from build123d import *

# Parameters (mm, degrees)
F2_R     = 1.5875
F3_DEPTH = 12.7
F4_SIZE  = 1.5875


with BuildPart() as f1:
    # F0 (on Front) → F1 (revolve)
    with BuildSketch(Plane.XZ):
        Polygon((1.27, 12.7), (0, 12.7), (-1.27, 12.7), (-1.27, 19.05), (-2.8575, 19.05), (-5.08, 6.35), (-5.08, 0), (5.08, 0), (5.08, 6.35), (2.8575, 19.05), (1.27, 19.05), align=None)
    revolve(axis=Axis((0, 0, 0), (-1, 0, 0)))

    # F2 (on Right) → F3 (cut, symmetric)
    with BuildSketch(Plane.YZ):
        Circle(F2_R)
    extrude(amount=F3_DEPTH, both=True, mode=Mode.SUBTRACT)

    # F4
    f4_edges = [f1.edges().sort_by_distance(p)[0] for p in [
        (5.08, -1.5875, 0),
        (-5.08, -1.5875, 0),
    ]]
    chamfer(f4_edges, length=F4_SIZE)


solid = f1.part
Geometry: final body of the model. Coordinates: model frame, mm. A direction names the side the tool comes from. Round coordinates to 2 decimals unless told otherwise and drop trailing zeros. Loops run counter-clockwise (first coordinate to the right, second up) from the corner with the lowest first, then second, coordinate; pieces in that order, holes last. Notation, with made-up numbers: M -18,68.5 L 6,68.5 A34 ccw 6,102.5 Z; hole C 71.25,30.25 d4. An arc over 180 degrees is marked long. Put each result on its own line as item: value. Start each with the question number.
(1) Material intervals for line 1 along X through (y, z) = (15, -11); line 2 along Z through (x, y) = (-0.5, -1); line 3 along X through (y, z) = (14.5, 4.5), sorted ascending. Write a range as [from, to].
(2) Section query C-C (x = -0.25). Return loops of the section in (y, z) (1 decimal).
(3) Draft query along X for faces 3 (the face through (-5.08, 3, -2)), 4 (the face through (-1.27, -4, -12.4)), 5 (the face through (4.94, -6.97, -1.55)), 6 (the face through (2.05, -11.59, -15.12)). Return one class per face: +X half, -X half, draft (parallel to the pull), parting line (faces both ways), or undercut.
(4) Set-up query: faces 1 (the face through (1.27, -4, 12.4)), 2 (the face through (-2.07, -11.59, -15.12)). Return all of +Z, -Z, +X, -X, +Y, -Y with unobstructed straight access to the full face (end or side cutting, diameter ignored); none if empty.
(5) Contact query for flat-ended pins moving along their axis: pin 1 Ø3.5 at (y, z) = (0, 0) entering from +X (3 decimals); pin 2 Ø4 at (x, y) = (3, -9.5) entering from +Z; pin 3 Ø10 at (y, z) = (4.5, -14.5) entering from -X. Output: stop coordinate, or through.
Findings below:
1. line 1: x = [-2.94, -1.27], [1.27, 2.94]
1. line 2: z = [-12.66, -1.23], [1.23, 12.66]
1. line 3: x = [-3.53, -1.27], [1.27, 3.53]
2. outline: C 0,0 d25.4; hole C 0,0 d3.2
3. face 3: -X half
3. face 4: undercut
3. face 5: +X half
3. face 6: draft
4. face 1: none
4. face 2: +X, -X
5. pin 1: stops at x = 3.655
5. pin 2: stops at z = 17.51
5. pin 3: stops at x = -4.41
